Geometry check sheet. Reference: the model listing, model coordinates, mm. Face numbers are marked on the shaded views. A direction names the side the tool comes from. Round coordinates to 2 decimals unless told otherwise and drop trailing zeros. Loops run counter-clockwise (first coordinate to the right, second up) from the corner with the lowest first, then second, coordinate; pieces in that order, holes last. Notation, with made-up numbers: (29, -19.5) -> (74, -19.5) arc R13 ccw to (74, -3.5) -> close; hole circle Ø8 at (-17, 56). An arc over 180 degrees is marked (long way). Use a Markdown table: item, result. Add a question column.
Q1. Sectioned sample at A-A, the plane y = 0. Enter the section's corners in (x, z), then the cut area to 3 significant figures.
Q2. Sectioned sample at B-B, the plane z = 3.45. Enter the section's corners in (x, y).
Q3. Set-up check for the marked faces 1, 2 and 3: record each of +Z, -Z, +X, -X, +Y, -Y from which the full face is reachable in a straight line by a thin tool's end or side.
Q4. Sectioned sample at D-D, the plane x = -16.5. Enter the section's corners in (y, z), then the cut area to 3 significant figures.
Q5. Sectioned sample at C-C, the plane y = 10.5. Enter the section's corners in (x, z), then the cut area to 3 significant figures.
Q6. Release check for a two-part mould opening along Y. For the marked faces 4, 5, 6 and 7 record: released by +Y, released by -Y, zero draft, split by the parting line, or undercut.
Q7. Material ranges on L1, parallel to X at y = 0, z = 3.3; L2, parallel to Y at x = 12.5, z = 4.55; L3, parallel to Y at x = 4.5, z = 4.3, recorded low to high.
Q8. Gauge pin test, flat ends, axial feed: P1, Ø1, axis at x = -15.5, y = -2, coming from the -Z side; P2, Ø2, axis at x = -12.63, y = 0, coming from the +Z side (3 decimals). Record the tip position at first contact, or that the pin passes through.
```python
from build123d import *

# Parameters (mm, degrees)
BOSS_EXTRUDE1_DEPTH     = 4.8
CUT_EXTRUDE1_DEPTH      = 31.859144724
CUT_EXTRUDE1_DEPTH_BACK = 31.859144724
CUT_EXTRUDE2_DEPTH      = 31.859144724
CUT_EXTRUDE2_DEPTH_BACK = 31.859144724
SKETCH1_13_R            = 1.25
CUT_EXTRUDE4_DEPTH      = 2.4
SKETCH2_W               = 5
SKETCH2_H               = 3.108471694
CUT_EXTRUDE5_DEPTH      = 31.859144724


with BuildPart() as part:
    # Sketch1 → Boss-Extrude1 (new body)
    with BuildSketch(Plane.XY):
        Polygon((-21.75, 18.25), (-21.75, -18.25), (-21.75, -21.358471694), (21.75, -21.358471694), (21.75, -18.25), (21.75, 18.25), (21.75, 21.358471694), (-21.75, 21.358471694), align=None)
    extrude(amount=BOSS_EXTRUDE1_DEPTH)

    # Sketch1_12 → Cut-Extrude1 (cut, two sides: drawn at the far end of the back side and taken through both)
    with BuildSketch(Plane.XY.offset(-CUT_EXTRUDE1_DEPTH_BACK)):
        Polygon((-7.25, 18.25), (-7.25, 4), (-7.25, 0), (-7.25, -4), (-7.25, -18.25), (7.25, -18.25), (7.25, -4), (7.25, 0), (7.25, 4), (7.25, 18.25), align=None)
    extrude(amount=CUT_EXTRUDE1_DEPTH + CUT_EXTRUDE1_DEPTH_BACK, mode=Mode.SUBTRACT)

    # Sketch1_13 → Cut-Extrude2 (cut, two sides: drawn at the far end of the back side and taken through both)
    with BuildSketch(Plane.XY.offset(-CUT_EXTRUDE2_DEPTH_BACK)):
        with Locations((-12.625438214, 0)):
            Circle(SKETCH1_13_R)
        with Locations((12.625438214, 0)):
            Circle(SKETCH1_13_R)
    extrude(amount=CUT_EXTRUDE2_DEPTH + CUT_EXTRUDE2_DEPTH_BACK, mode=Mode.SUBTRACT)

    # Sketch1_15 → Cut-Extrude4 (cut)
    with BuildSketch(Plane.XY):
        with BuildLine():
            Line((-7.25, 4), (-19.25, 4))
            Line((-19.25, 4), (-19.25, 0))
            Line((-19.25, 0), (-13.875438214, 0))
            ThreePointArc((-13.875438214, 0), (-12.625438214, 1.25), (-11.375438214, 0))
            Line((-11.375438214, 0), (-7.25, 0))
            Line((-7.25, 0), (-7.25, 4))
        make_face()
        with BuildLine():
            Line((-13.875438214, 0), (-19.25, 0))
            Line((-19.25, 0), (-19.25, -4))
            Line((-19.25, -4), (-7.25, -4))
            Line((-7.25, -4), (-7.25, 0))
            Line((-7.25, 0), (-11.375438214, 0))
            ThreePointArc((-11.375438214, 0), (-12.625438214, -1.25), (-13.875438214, 0))
        make_face()
        with BuildLine():
            Line((19.25, 4), (7.25, 4))
            Line((7.25, 4), (7.25, 0))
            Line((7.25, 0), (11.375438214, 0))
            ThreePointArc((11.375438214, 0), (12.625438214, 1.25), (13.875438214, 0))
            Line((13.875438214, 0), (19.25, 0))
            Line((19.25, 0), (19.25, 4))
        make_face()
        with BuildLine():
            Line((11.375438214, 0), (7.25, 0))
            Line((7.25, 0), (7.25, -4))
            Line((7.25, -4), (19.25, -4))
            Line((19.25, -4), (19.25, 0))
            Line((19.25, 0), (13.875438214, 0))
            ThreePointArc((13.875438214, 0), (12.625438214, -1.25), (11.375438214, 0))
        make_face()
    extrude(amount=CUT_EXTRUDE4_DEPTH, mode=Mode.SUBTRACT)

    # Sketch2 → Cut-Extrude5 (cut, through all)
    with BuildSketch(Plane(origin=(0, 0, 0), x_dir=(-1, 0, 0), z_dir=(0, 0, -1))):
        with Locations((0, -19.804235847)):
            Rectangle(SKETCH2_W, SKETCH2_H)
    extrude(amount=-CUT_EXTRUDE5_DEPTH, mode=Mode.SUBTRACT)


solid = part.part
```
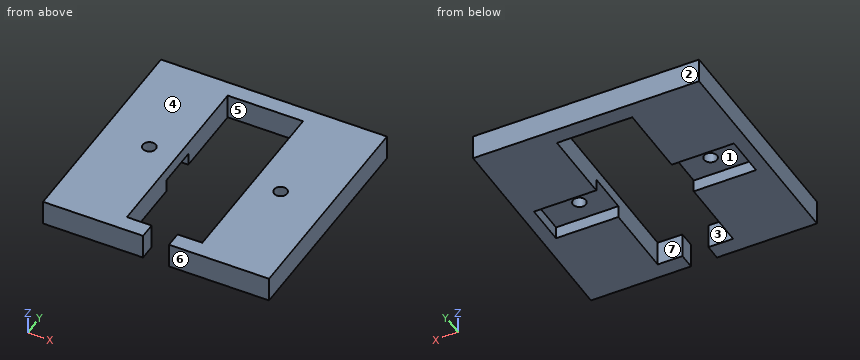
Values:
| question | item | result |
|---|---|---|
| 1 | outline | (-21.75, 0) -> (-19.25, 0) -> (-19.25, 2.4) -> (-13.88, 2.4) -> (-13.88, 4.8) -> (-21.75, 4.8) -> close; (-11.38, 2.4) -> (-7.25, 2.4) -> (-7.25, 4.8) -> (-11.38, 4.8) -> close; (7.25, 2.4) -> (11.38, 2.4) -> (11.38, 4.8) -> (7.25, 4.8) -> close; (13.88, 2.4) -> (19.25, 2.4) -> (19.25, 0) -> (21.75, 0) -> (21.75, 4.8) -> (13.88, 4.8) -> close |
| 1 | area | 69.6 mm^2 |
| 2 | outline | (-21.75, -21.36) -> (-2.5, -21.36) -> (-2.5, -18.25) -> (-7.25, -18.25) -> (-7.25, 18.25) -> (7.25, 18.25) -> (7.25, -18.25) -> (2.5, -18.25) -> (2.5, -21.36) -> (21.75, -21.36) -> (21.75, 21.36) -> (-21.75, 21.36) -> close; hole circle Ø2.5 at (-12.63, 0); hole circle Ø2.5 at (12.63, 0) |
| 3 | face 1 | -Z |
| 3 | face 2 | +Z, -Z, +X, -X, +Y |
| 3 | face 3 | +Z, -Z |
| 4 | outline | (-21.36, 0) -> (-4, 0) -> (-4, 2.4) -> (4, 2.4) -> (4, 0) -> (21.36, 0) -> (21.36, 4.8) -> (-21.36, 4.8) -> close |
| 4 | area | 186 mm^2 |
| 5 | outline | (-21.75, 0) -> (-7.25, 0) -> (-7.25, 4.8) -> (-21.75, 4.8) -> close; (7.25, 0) -> (21.75, 0) -> (21.75, 4.8) -> (7.25, 4.8) -> close |
| 5 | area | 139 mm^2 |
| 6 | face 4 | zero draft |
| 6 | face 5 | undercut |
| 6 | face 6 | released by -Y |
| 6 | face 7 | undercut |
| 7 | L1 | -21.75 to -13.88, -11.38 to -7.25, 7.25 to 11.38, 13.88 to 21.75 |
| 7 | L2 | -21.36 to -1.24, 1.24 to 21.36 |
| 7 | L3 | -21.36 to -18.25, 18.25 to 21.36 |
| 8 | P1 | z = 2.4 |
| 8 | P2 | through |
